Drawing for the job (mm, zero at the part's lowest x, y, z). A direction names the side the tool comes from. Round coordinates to 2 decimals unless told otherwise and drop trailing zeros. Loops run counter-clockwise (first coordinate to the right, second up) from the corner with the lowest first, then second, coordinate; pieces in that order, holes last. Notation, with made-up numbers: M 28,35 L 46,35 A20 ccw 46,74 Z; hole C 27,63 d10. An arc over 180 degrees is marked long. Write each question's results on one line, items separated by ' | '.
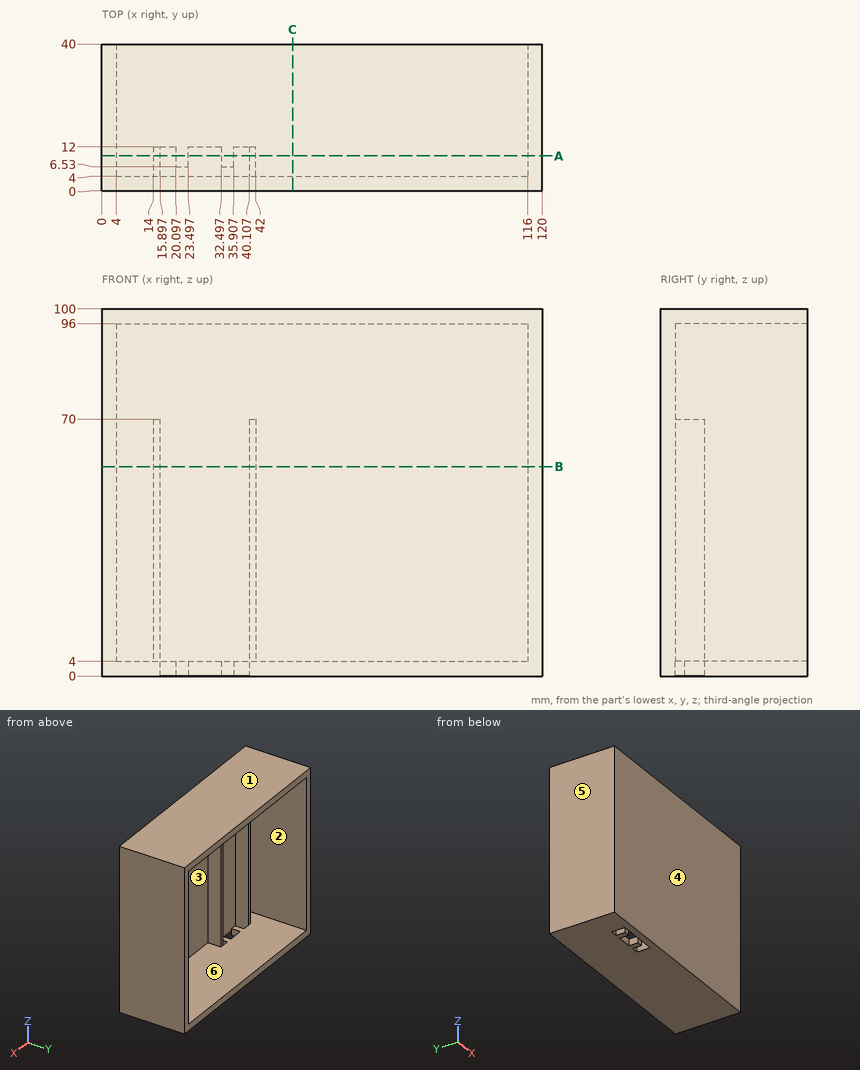
Item 1: Which spindle directions (+Z, -Z, +X, -X, +Y, -Y) get a long thin tool onto all of the face, cutting with end or side? Do the marked faces 5 and 6. Say none if no direction does.
Filled sheet:
face 5: +Z, -Z, -X, +Y, -Y | face 6: +Y
Item 2: Drop flat-ended pins along their axis: P1, Ø2, axis at x = 27, z = 3, coming from the -Y side; P2, Ø2, axis at x = 41, z = 41, coming from the +Y side. Give the stop position or say it passes through.
Filled sheet:
P1: y = 0 | P2: y = 12
Item 3: Band-saw the part on C-C on x = 52. Give the cut face in (y, z), and give its area (3 significant figures).
Filled sheet:
outline: M 0,0 L 40,0 L 40,4 L 4,4 L 4,96 L 40,96 L 40,100 L 0,100 Z | area: 688 mm^2
Item 4: Two-plate mould, pull along Z, no slides. Class the marked faces 1, 2, 3 and 4: +Z half, -Z half, draft (parallel to the pull), parting line (faces both ways), or undercut.
Filled sheet:
face 1: +Z half | face 2: undercut | face 3: undercut | face 4: draft
Item 5: Wall check: L1, parallel to X at y = 5.5, z = 24; L2, parallel to X at y = 24.5, z = 26; L3, parallel to Z at x = 24, y = 23.5. Give the ranges that are in metal, low to high.
Filled sheet:
L1: 0 to 4, 14 to 15.9, 40.11 to 42, 116 to 120 | L2: 0 to 4, 116 to 120 | L3: 0 to 4, 96 to 100
Item 6: Band-saw the part on A-A on y = 9.5. Give the cut face in (x, z).
Filled sheet:
outline: M 0,0 L 15.9,0 L 15.9,70 L 14,70 L 14,4 L 4,4 L 4,96 L 116,96 L 116,4 L 42,4 L 42,70 L 40.11,70 L 40.11,0 L 120,0 L 120,100 L 0,100 Z; M 20.1,0 L 23.5,0 L 23.5,4 L 20.1,4 Z; M 32.5,0 L 35.91,0 L 35.91,4 L 32.5,4 Z
Item 7: Band-saw the part on B-B on z = 57. Give the cut face in (x, y).
Filled sheet:
outline: M 0,0 L 120,0 L 120,40 L 116,40 L 116,4 L 42,4 L 42,12 L 40.11,12 L 40.11,4 L 15.9,4 L 15.9,12 L 14,12 L 14,4 L 4,4 L 4,40 L 0,40 Z
